Check sheet for the modelled part. Datum: model origin and axes. Units: mm. Face numbers are marked on the shaded views. A direction names the side the tool comes from. Round coordinates to 2 decimals unless told otherwise and drop trailing zeros. Write each loop counter-clockwise with the first axis right and the second up, starting at its lowest first coordinate (ties: lowest second). Pieces come first, ordered by that corner, then holes.
Item 1: Depth check by flat-ended pin: pin 1 (3 mm diameter, centred on x = 1.5, z = 7.5, fed in from +Y). Enter the tip coordinate at first touch or a pass-through.
Item 2: Set-up check for the marked faces 1 and 2: record each of +Z, -Z, +X, -X, +Y, -Y from which the full face is reachable in a straight line by a thin tool's end or side.
Item 3: Section check B-B, the plane z = 4. Record the cut outline in (x, y).
Item 4: Release check for a two-part mould opening along Y. For the marked faces 3, 4 and 5 record: pulls with the +Y half, pulls with the -Y half, needs draft (parallel to the pull), parting line crosses it, or undercut.
Item 5: Section check A-A, the plane x = 0. Record the cut outline in (y, z).
Item 6: Material ranges on line 1 along X through (y, z) = (-0.1, 10); line 2 along Y through (x, z) = (0.55, 13); line 3 along Z through (x, y) = (-0.1, -0.6), recorded low to high.
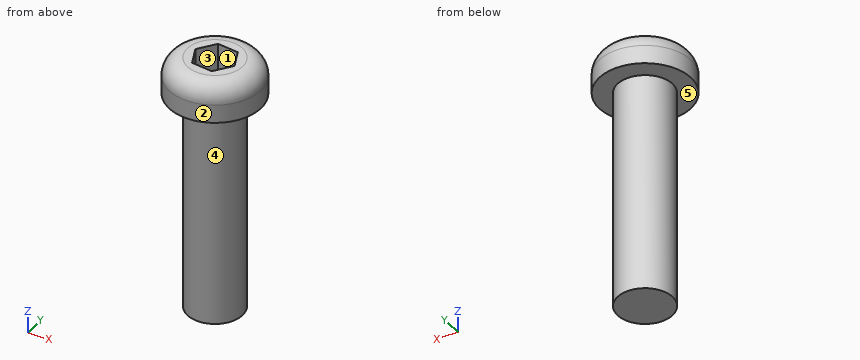
from build123d import *

# Parameters (mm, degrees)
SKETCH_1_R          = 1.5
EXTRUDE_1_DEPTH     = 12
SKETCH_2_R          = 2.5
EXTRUDE_2_DEPTH     = 2
CUT_EXTRUDE_1_DEPTH = 1.5
FILLET_2_R          = 1


with BuildPart() as part:
    # 草图1 → 凸台-拉伸1 (new body)
    with BuildSketch(Plane.XY):
        Circle(SKETCH_1_R)
    extrude(amount=EXTRUDE_1_DEPTH)

    # 草图2 → 凸台-拉伸2 (add)
    with BuildSketch(Plane.XY.offset(12)):
        Circle(SKETCH_2_R)
    extrude(amount=EXTRUDE_2_DEPTH)

    # 草图3 → 切除-拉伸1 (cut)
    with BuildSketch(Plane.XY.offset(14)):
        Polygon((1.149641735, -0.107968584), (0.668324404, 0.941634655), (-0.481317331, 1.04960324), (-1.149641735, 0.107968584), (-0.668324404, -0.941634655), (0.481317331, -1.04960324), align=None)
    extrude(amount=-CUT_EXTRUDE_1_DEPTH, mode=Mode.SUBTRACT)

    # 圆角2
    fillet_2_edges = [part.edges().sort_by_distance(p)[0] for p in [
        (-2.5, 0, 14),
    ]]
    fillet(fillet_2_edges, radius=FILLET_2_R)


solid = part.part
Values found:
1. pin 1: stops at y = 1.5
2. face 1: +Z
2. face 2: +Z, -Z
3. outline: circle Ø3 at (0, 0)
4. face 3: undercut
4. face 4: parting line crosses it
4. face 5: needs draft
5. outline: (-2.5, 12) - (-1.5, 12) - (-1.5, 0) - (1.5, 0) - (1.5, 12) - (2.5, 12) - (2.5, 13) arc R1 ccw to (1.5, 14) - (1, 14) - (1, 12.5) - (-1, 12.5) - (-1, 14) - (-1.5, 14) arc R1 ccw to (-2.5, 13) - close
6. line 1: x = -1.5 to 1.5
6. line 2: y = -2.44 to -0.95, 0.95 to 2.44
6. line 3: z = 0 to 12.5
